The listing builds one solid part. Answer for the finished solid, in the listing's coordinates (mm). A direction names the side the tool comes from. Coordinates: 2 decimals unless noted, no trailing zeros. Write each loop counter-clockwise with the first axis right and the second up, starting at its lowest first coordinate (ties: lowest second). Pieces come first, ordered by that corner, then holes.
(1) The part is cut by section A-A on z = 2. Determine the outline of the cut face in (x, y).
(2) Which of the six approach directions +Z, -Z, +X, -X, +Y, -Y give full straight-line access (tool end or side, diameter ignored) to faces 5 (the flat face through (106, 33.305, 10)), 6 (the flat face through (83.253, 60, 15)), 7 (the flat face through (20, 71.11, 10)), 8 (the flat face through (40, 19.566, 10))?
(3) For a pull along X with two mould halves and no side action, classify faces 1 (the flat face through (40, 47.185, 10)), 2 (the flat face through (38.886, 86, 10)), 3 (the flat face through (107.489, 70, 15)), 4 (the flat face through (125, 66, 10)) as +X half, -X half, draft (parallel to the pull), parting line (faces both ways), or undercut.
(4) The part is cut by section D-D on z = 15. Determine the outline of the cut face in (x, y), plus the area to 3 significant figures.
(5) The part is cut by section C-C on y = 43.5. Determine the outline of the cut face in (x, z), plus the area to 3 significant figures.
(6) The part is cut by section B-B on x = 47. Determine the outline of the cut face in (y, z).
(7) Given P1, Ø10, axis at x = 42, y = 57.5, coming from the -Z side; P2, Ø3, axis at y = 77, z = 13.5, coming from the -X side; P3, Ø2, axis at x = 96.5, y = 72, coming from the +Z side; P4, Ø3, axis at x = 90, z = 10.5, coming from the -Y side, each flat-ended and moving along its own axis, determine where each tip first touches the part or whether it passes through.
(8) Straight lines are drawn through the part: line 1 (X direction, y = 69.5, z = 10.5); line 2 (Y direction, x = 31.5, z = 16); line 3 (Y direction, x = 47, z = 9). For each, find the intervals that lie inside material, in ascending order.
from build123d import *

# Parameters (mm, degrees)
EXTRUDE1_DEPTH     = 20
SKETCH2_W          = 36.686074526
SKETCH2_H          = 27.619463242
CUT_EXTRUDE1_DEPTH = 20
CUT_EXTRUDE2_DEPTH = 10


with BuildPart() as part:
    # Sketch1 → Extrude1 (new body)
    with BuildSketch(Plane.XY):
        Polygon((0, 0), (87.492525773, 0), (87.492525773, 33.304768041), (125, 33.304768041), (125, 100), (38.88556701, 100), (38.88556701, 71.110180412), (0, 71.110180412), align=None)
    extrude(amount=EXTRUDE1_DEPTH)

    # Sketch2 → Cut-Extrude1 (cut)
    with BuildSketch(Plane.XY.offset(20)):
        with Locations((39.952253424, 33.375570886)):
            Rectangle(SKETCH2_W, SKETCH2_H)
    extrude(amount=-CUT_EXTRUDE1_DEPTH, mode=Mode.SUBTRACT)

    # Sketch3 → Cut-Extrude2 (cut)
    with BuildSketch(Plane.XY.offset(20)):
        Polygon((60.658966885, 88.995285907), (107.488557574, 88.995285907), (107.488557574, 50.5688125), (83.253213497, 50.5688125), (83.253213497, 69.608647213), (60.658966885, 69.608647213), align=None)
    extrude(amount=-CUT_EXTRUDE2_DEPTH, mode=Mode.SUBTRACT)


solid = part.part
Model answer:
1. outline: (0, 0) - (87.49, 0) - (87.49, 33.3) - (125, 33.3) - (125, 100) - (38.89, 100) - (38.89, 71.11) - (0, 71.11) - close; hole (21.61, 19.57) - (58.3, 19.57) - (58.3, 47.19) - (21.61, 47.19) - close
2. face 5: +Z, -Z, +X, -Y
2. face 6: +Z
2. face 7: +Z, -Z, -X, +Y
2. face 8: +Z, -Z
3. face 1: undercut
3. face 2: -X half
3. face 3: undercut
3. face 4: +X half
4. outline: (0, 0) - (87.49, 0) - (87.49, 33.3) - (125, 33.3) - (125, 100) - (38.89, 100) - (38.89, 71.11) - (0, 71.11) - close; hole (21.61, 19.57) - (58.3, 19.57) - (58.3, 47.19) - (21.61, 47.19) - close; hole (60.66, 69.61) - (83.25, 69.61) - (83.25, 50.57) - (107.49, 50.57) - (107.49, 89) - (60.66, 89) - close
4. area: 7,740 mm2
5. outline: (0, 0) - (21.61, 0) - (21.61, 20) - (0, 20) - close; (58.3, 0) - (125, 0) - (125, 20) - (58.3, 20) - close
5. area: 1,770 mm2
6. outline: (0, 0) - (19.57, 0) - (19.57, 20) - (0, 20) - close; (47.19, 0) - (100, 0) - (100, 20) - (47.19, 20) - close
7. P1: stops at z = 0
7. P2: stops at x = 38.89
7. P3: stops at z = 10
7. P4: stops at y = 33.3
8. line 1: x = 0 to 83.25, 107.49 to 125
8. line 2: y = 0 to 19.57, 47.19 to 71.11
8. line 3: y = 0 to 19.57, 47.19 to 100
